```python
from build123d import *

# Parameters (mm, degrees)
F0_W     = 63.5
F0_H     = 38.1
F1_DEPTH = 3.175
F2_W     = 6.35
F2_H     = 3.175
F3_DEPTH = 6.35
F4_R     = 1.5875
F5_DEPTH = 25.4


with BuildPart() as f1:
    # F0 (on Top) → F1 (new body)
    with BuildSketch(Plane.XY):
        with Locations((25.302306, 74.666583)):
            Rectangle(F0_W, F0_H)
    extrude(amount=F1_DEPTH)

    # F2 (on face) → F3 (join)
    with BuildSketch(Plane.YZ.offset(57.052306)):
        with Locations((58.791583, 1.5875)):
            Rectangle(F2_W, F2_H)
        with Locations((90.541583, 1.5875)):
            Rectangle(F2_W, F2_H)
    extrude(amount=F3_DEPTH)

    # F4 (on face) → F5 (join)
    with BuildSketch(Plane(origin=(0, 61.966583, 0), x_dir=(-1, 0, 0), z_dir=(0, 1, 0))):
        with Locations((-61.497306, 1.5875)):
            Circle(F4_R)
    extrude(amount=F5_DEPTH)


solid = f1.part
```
Verification items for the finished model (mm, model axes). A direction names the side the tool comes from. Give positions to 0.01 mm unless a question says otherwise; leave off trailing zeros. Order: outer loops, then holes, each group sorted by start corner. A loop starts at its lowest first (then second) coordinate and runs counter-clockwise, first axis right, second up. Notation, with made-up numbers: M 25,64.25 L 38,64.25 A35 ccw 38,96.25 Z; hole C 68,38 d2. An arc over 180 degrees is marked long. Answer in a Markdown table with one row per item. Add a question column.
Item 1: Tool access check on faces 4 (the flat face through (57.052, 74, 2)), 5 (the flat face through (63.22, 87.367, 1.82)), 6 (the flat face through (63.402, 90, 2)). Record the directions out of +Z, -Z, +X, -X, +Y, -Y that give a thin tool (end or side, any length) a straight path to the whole face; none if there is none.
Item 2: Gauge pin test, flat end, axial feed: pin 1 (1 mm diameter, centred on y = 70.5, z = 1, fed in from +X). Record the tip position at first contact, or that the pin passes through.
Item 3: Section check A-A, the plane z = 2.1. Enter the section's corners in (x, y), and give its area (3 significant figures).
Item 4: Mould release check, pull along X, two halves, no side actions. Record for faces 1 (the flat face through (63.402, 59, 2)), 2 (the flat face through (28, 74, 3.175)), 3 (the cylindrical face through (59.98, 74.49, 2.06)): released by +X, released by -X, zero draft, split by the parting line, or undercut.
Item 5: Section check B-B, the plane y = 76. Enter the section's corners in (x, z) (1 decimal), and give its area (3 significant figures).
Item 6: Scan lines: probe 1 along X at (y, z) = (66, 1.4); probe 2 along X at (y, z) = (68, 0.8). Record each from-to range of solid material in increasing order. Write a range as from..to.
Filled sheet:
| question | item | result |
|---|---|---|
| 1 | face 4 | +Z, -Z |
| 1 | face 5 | +X |
| 1 | face 6 | +Z, -Z, +X, +Y, -Y |
| 2 | pin 1 | stops at x = 63.08 |
| 3 | outline | M -6.45,55.62 L 63.4,55.62 L 63.4,61.97 L 63,61.97 L 63,87.37 L 63.4,87.37 L 63.4,93.72 L -6.45,93.72 Z; hole M 57.05,61.97 L 59.99,61.97 L 59.99,87.37 L 57.05,87.37 Z |
| 3 | area | 2,580 mm^2 |
| 4 | face 1 | released by +X |
| 4 | face 2 | zero draft |
| 4 | face 3 | undercut |
| 5 | outline | M -6.4,0 L 57.1,0 L 57.1,3.2 L -6.4,3.2 Z; C 61.5,1.6 d3.2 |
| 5 | area | 210 mm^2 |
| 6 | probe 1 | x = -6.45..57.05, 59.92..63.07 |
| 6 | probe 2 | x = -6.45..57.05, 60.12..62.88 |
